The model under review builds one solid part; all positions refer to its coordinate system, in mm. Face numbers are marked on the shaded views. A direction names the side the tool comes from. Round coordinates to 2 decimals unless told otherwise and drop trailing zeros. Loops run counter-clockwise (first coordinate to the right, second up) from the corner with the lowest first, then second, coordinate; pieces in that order, holes last. Notation, with made-up numbers: (57, 77.25) -> (87, 77.25) arc R25 cw to (87, 99.25) -> close; hole circle Ø9 at (43, 85.25). An arc over 180 degrees is marked (long way). Use CSV: the item, a comma, the result in double quotes. Start each with the question number.
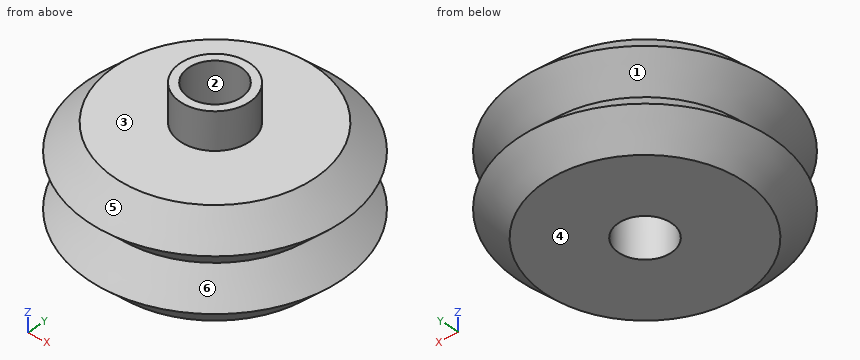
Solid Edge part; units mm, degrees
sketch "Sketch1" plane through (0, 0, 0) normal (0, -1, 0) x (1, 0, 0)
  line L0 (12, 2.55) -> (9.45, 5.1)
  line L1 (0, 5.1) -> (9.45, 5.1)
  line L2 (0, 0) -> (0, 5.1)
  line L3 (0, 0) -> (0, -5.1)
  line L4 (0, -5.1) -> (9.45, -5.1)
  line L5 (12, -2.55) -> (9.45, -5.1)
  line L6 (12, -2.55) -> (9.45, 0)
  line L7 (12, 2.55) -> (9.45, 0)
revolve "RevolvedProtrusion1" add sketch "Sketch1" angle 360 about axis through (0, 0, 0) along (0, 0, -1)
sketch "Sketch2" plane through (0, 0, 5.1) normal (0, 0, 1) x (1, 0, 0)
  circle A0 centre (0, 0) radius 2.5
extrude "Cutout1" cut sketch "Sketch2" against normal up to vertex (10.2 mm away)
sketch "Sketch3" plane through (0, 0, 5.1) normal (0, 0, 1) x (1, 0, 0)
  circle A0 centre (0, 0) radius 3.284
  circle A1 centre (0, 0) radius 2.5
extrude "Protrusion1" add sketch "Sketch3" along normal blind 3.5
1. Take a section at A-A, the plane y = 0. Give the boundary of the cut face in (x, z), then the cut area to 3 significant figures.
2. The part is to be moulded in two halves that separate along Z. For the marked faces 4, 5 and 6, say which applies: pulls with the +Z half, pulls with the -Z half, needs draft (parallel to the pull), parting line crosses it, or undercut.
3. For line 1 along Z through (x, y) = (1, -5.5); line 2 along Z through (x, y) = (6.5, -8); line 3 along Z through (x, y) = (10, -4), list the stretches that pass through material, from the lowest coordinate up. Write a range as from..to.
4. Take a section at D-D, the plane z = -1.25. Give the boundary of the cut face in (x, y).
5. Clearance check with flat-ended pins moving along their axes: P1, Ø2, axis at x = 9, z = 0.5, coming from the -Y side; P2, Ø1, axis at x = -5, z = -3.5, coming from the +Y side; P3, Ø6, axis at x = -7, z = -3, coming from the +Y side; P4, Ø6.5, axis at x = 0, y = 0, coming from the +Z side. State where each tip first meets the part, or that it passes through.
6. Take a section at C-C, the plane z = 1. Give the boundary of the cut face in (x, y), then the cut area to 3 significant figures.
7. For the marked faces 1, 2 and 3, list the 3-axis set-ups (+Z, -Z, +X, -X, +Y, -Y) from which the entire face can be reached by the end or side of a thin tool; tool diameter is ignored.
Results:
1,outline,"(-12, -2.55) -> (-9.45, -5.1) -> (-2.5, -5.1) -> (-2.5, 8.6) -> (-3.28, 8.6) -> (-3.28, 5.1) -> (-9.45, 5.1) -> (-12, 2.55) -> (-9.45, 0) -> close; (2.5, -5.1) -> (9.45, -5.1) -> (12, -2.55) -> (9.45, 0) -> (12, 2.55) -> (9.45, 5.1) -> (3.28, 5.1) -> (3.28, 8.6) -> (2.5, 8.6) -> close"
1,area,"173 mm²"
2,face 4,"pulls with the -Z half"
2,face 5,"pulls with the +Z half"
2,face 6,"undercut"
3,line 1,"-5.1..5.1"
3,line 2,"-4.24..-0.86, 0.86..4.24"
3,line 3,"-3.78..-1.32, 1.32..3.78"
4,outline,"circle Ø21.4 at (0, 0); hole circle Ø5 at (0, 0)"
5,P1,"y = -6.71"
5,P2,"y = 10.46"
5,P3,"y = 11.3"
5,P4,"z = 8.6"
6,outline,"circle Ø20.9 at (0, 0); hole circle Ø5 at (0, 0)"
6,area,"323 mm²"
7,face 1,"none"
7,face 2,"+Z, -Z"
7,face 3,"+Z"
